Geometry check sheet. Reference: the model listing, model coordinates, mm. A direction names the side the tool comes from. Round coordinates to 2 decimals unless told otherwise and drop trailing zeros. Order: outer loops, then holes, each group sorted by start corner. A loop starts at its lowest first (then second) coordinate and runs counter-clockwise, first axis right, second up.
```python
from build123d import *

# Parameters (mm, degrees)
SKETCH_2_W            = 30
SKETCH_2_H            = 30
EXTRUDE_9_DEPTH       = 2
SKETCH_5_R            = 6.5
SKETCH_5_R_2          = 1.44
EXTRUDE_11_DEPTH      = 9.7
SKETCH_2_17_W         = 30
SKETCH_2_17_H         = 30
EXTRUDE_12_DEPTH      = 3.5
SKETCH_5_4_R          = 6.5
SKETCH_5_4_R_2        = 1.44
EXTRUDE_13_DEPTH      = 10
EXTRUDE_17_DEPTH      = 10
EXTRUDE_17_DEPTH_BACK = 2
SKETCH_5_8_R          = 6.5
SKETCH_5_8_R_2        = 1.44
SKETCH_5_11_R         = 6.5
SKETCH_5_11_R_2       = 1.44
EXTRUDE_18_DEPTH      = 13
SKETCH_2_18_W         = 30
SKETCH_2_18_H         = 30
EXTRUDE_19_DEPTH      = 3
SKETCH_6_R            = 1.45
CUT_EXTRUDE_1_DEPTH   = 3.5


with BuildPart() as part:
    # Sketch 2 → Extrude 9 (new body)
    with BuildSketch(Plane.XY):
        with BuildLine():
            Line((15, -15), (15, 15))
            ThreePointArc((15, 15), (30, 0), (15, -15))
        make_face()
        with BuildLine():
            Line((-15, 15), (15, 15))
            ThreePointArc((15, 15), (0, 30), (-15, 15))
        make_face()
        with BuildLine():
            Line((-15, -15), (-15, 15))
            ThreePointArc((-15, 15), (-30, 0), (-15, -15))
        make_face()
        with BuildLine():
            Line((-15, -15), (15, -15))
            ThreePointArc((15, -15), (0, -30), (-15, -15))
        make_face()
        Rectangle(SKETCH_2_W, SKETCH_2_H)
    extrude(amount=EXTRUDE_9_DEPTH)

    # Sketch 5 → Extrude 11 (add)
    # profile 1 of 2: a face of its own
    with BuildSketch(Plane.XY.offset(2)):
        with Locations((-15, 0)):
            Circle(SKETCH_5_R)
        with Locations((-15, 0)):
            Circle(SKETCH_5_R_2, mode=Mode.SUBTRACT)
    # profile 2 of 2: a face of its own
    with BuildSketch(Plane.XY.offset(2)):
        with Locations((15, 0)):
            Circle(SKETCH_5_R)
        with Locations((15, 0)):
            Circle(SKETCH_5_R_2, mode=Mode.SUBTRACT)
    extrude(amount=EXTRUDE_11_DEPTH)

    # Sketch 2_17 → Extrude 12 (add)
    with BuildSketch(Plane.XY):
        with BuildLine():
            Line((-15, 15), (15, 15))
            ThreePointArc((15, 15), (0, 30), (-15, 15))
        make_face()
        Rectangle(SKETCH_2_17_W, SKETCH_2_17_H)
        with BuildLine():
            Line((-15, -15), (15, -15))
            ThreePointArc((15, -15), (0, -30), (-15, -15))
        make_face()
        with BuildLine():
            Line((15, -15), (15, 15))
            ThreePointArc((15, 15), (30, 0), (15, -15))
        make_face()
        with BuildLine():
            Line((-15, -15), (-15, 15))
            ThreePointArc((-15, 15), (-30, 0), (-15, -15))
        make_face()
    extrude(amount=EXTRUDE_12_DEPTH)

    # Sketch 5_4 → Extrude 13 (add)
    # profile 1 of 2: a face of its own
    with BuildSketch(Plane.XY.offset(2)):
        with Locations((-15, 0)):
            Circle(SKETCH_5_4_R)
        with Locations((-15, 0)):
            Circle(SKETCH_5_4_R_2, mode=Mode.SUBTRACT)
    # profile 2 of 2: a face of its own
    with BuildSketch(Plane.XY.offset(2)):
        with Locations((15, 0)):
            Circle(SKETCH_5_4_R)
        with Locations((15, 0)):
            Circle(SKETCH_5_4_R_2, mode=Mode.SUBTRACT)
    extrude(amount=EXTRUDE_13_DEPTH)

    # Sketch 5_8 → Extrude 17 (add, two sides: drawn at the far end of the back side and taken through both)
    # profile 1 of 2: a face of its own
    with BuildSketch(Plane.XY.offset(2).offset(-EXTRUDE_17_DEPTH_BACK)):
        with Locations((-15, 0)):
            Circle(SKETCH_5_8_R)
        with Locations((-15, 0)):
            Circle(SKETCH_5_8_R_2, mode=Mode.SUBTRACT)
    # profile 2 of 2: a face of its own
    with BuildSketch(Plane.XY.offset(2).offset(-EXTRUDE_17_DEPTH_BACK)):
        with Locations((15, 0)):
            Circle(SKETCH_5_8_R)
        with Locations((15, 0)):
            Circle(SKETCH_5_8_R_2, mode=Mode.SUBTRACT)
    extrude(amount=EXTRUDE_17_DEPTH + EXTRUDE_17_DEPTH_BACK)

    # Sketch 5_11 → Extrude 18 (add)
    # profile 1 of 2: a face of its own
    with BuildSketch(Plane.XY.offset(2)):
        with Locations((-15, 0)):
            Circle(SKETCH_5_11_R)
        with Locations((-15, 0)):
            Circle(SKETCH_5_11_R_2, mode=Mode.SUBTRACT)
    # profile 2 of 2: a face of its own
    with BuildSketch(Plane.XY.offset(2)):
        with Locations((15, 0)):
            Circle(SKETCH_5_11_R)
        with Locations((15, 0)):
            Circle(SKETCH_5_11_R_2, mode=Mode.SUBTRACT)
    extrude(amount=EXTRUDE_18_DEPTH)

    # Sketch 2_18 → Extrude 19 (add)
    with BuildSketch(Plane.XY):
        with BuildLine():
            Line((-15, 15), (15, 15))
            ThreePointArc((15, 15), (0, 30), (-15, 15))
        make_face()
        Rectangle(SKETCH_2_18_W, SKETCH_2_18_H)
        with BuildLine():
            Line((-15, -15), (-15, 15))
            ThreePointArc((-15, 15), (-30, 0), (-15, -15))
        make_face()
        with BuildLine():
            Line((15, -15), (15, 15))
            ThreePointArc((15, 15), (30, 0), (15, -15))
        make_face()
        with BuildLine():
            Line((-15, -15), (15, -15))
            ThreePointArc((15, -15), (0, -30), (-15, -15))
        make_face()
    extrude(amount=EXTRUDE_19_DEPTH)

    # Sketch 6 → Cut-Extrude 1 (cut)
    with BuildSketch(Plane.XY.offset(3.5)):
        with Locations((0, 26)):
            Circle(SKETCH_6_R)
        with Locations((-26, 0)):
            Circle(SKETCH_6_R)
        with Locations((26, 0)):
            Circle(SKETCH_6_R)
        with Locations((0, -26)):
            Circle(SKETCH_6_R)
    extrude(amount=-CUT_EXTRUDE_1_DEPTH, mode=Mode.SUBTRACT)


solid = part.part
```
(1) Depth check by flat-ended pin: P1, Ø3, axis at x = 21.5, z = 4, coming from the +Y side; P2, Ø8, axis at x = -17.5, z = 13, coming from the +Y side; P3, Ø1.7, axis at x = 0, y = 26, coming from the -Z side; P4, Ø5, axis at y = 4, z = 11, coming from the -X side. Enter the tip coordinate at first touch or a pass-through.
Returned:
P1: stops at y = 14.11
P2: stops at y = 6.5
P3: passes through
P4: stops at x = -21.32
(2) Sectioned sample at B-B, the plane z = 8.75. Record the cut outline in (x, y).
Returned:
outline: circle Ø13 at (-15, 0); circle Ø13 at (15, 0); hole circle Ø2.88 at (-15, 0); hole circle Ø2.88 at (15, 0)
(3) Material ranges on line 1 (X direction, y = 0, z = 7.25); line 2 (Y direction, x = 0, z = 1.55); line 3 (Y direction, x = 15, z = 12), recorded low to high.
Returned:
line 1: x = -21.5 to -16.44, -13.56 to -8.5, 8.5 to 13.56, 16.44 to 21.5
line 2: y = -30 to -27.45, -24.55 to 24.55, 27.45 to 30
line 3: y = -6.5 to -1.44, 1.44 to 6.5
(4) Set-up check for faces 5 (the cylindrical face through (-13.67, -0.55, 9.17)), 6 (the cylindrical face through (-0.314, 24.584, 1.774)): record each of +Z, -Z, +X, -X, +Y, -Y from which the full face is reachable in a straight line by a thin tool's end or side.
Returned:
face 5: +Z
face 6: +Z, -Z
(5) Draft check along Y on faces 1 (the cylindrical face through (16.33, -0.55, 9.17)), 2 (the cylindrical face through (-21.494, 0.286, 9.17)), 3 (the cylindrical face through (0, -30, 2)), 4 (the flat face through (0, 0, 3.5)). Enter one of: released by +Y, released by -Y, zero draft, split by the parting line, or undercut.
Returned:
face 1: undercut
face 2: split by the parting line
face 3: released by -Y
face 4: zero draft
(6) Sectioned sample at A-A, the plane x = 0. Record the cut outline in (y, z).
Returned:
outline: (-30, 0) - (-27.45, 0) - (-27.45, 3.5) - (-30, 3.5) - close; (-24.55, 0) - (24.55, 0) - (24.55, 3.5) - (-24.55, 3.5) - close; (27.45, 0) - (30, 0) - (30, 3.5) - (27.45, 3.5) - close
(7) Sectioned sample at C-C, the plane x = -26. Record the cut outline in (y, z).
Returned:
outline: (-10.2, 0) - (-1.45, 0) - (-1.45, 3.5) - (-10.2, 3.5) - close; (1.45, 0) - (10.2, 0) - (10.2, 3.5) - (1.45, 3.5) - close
